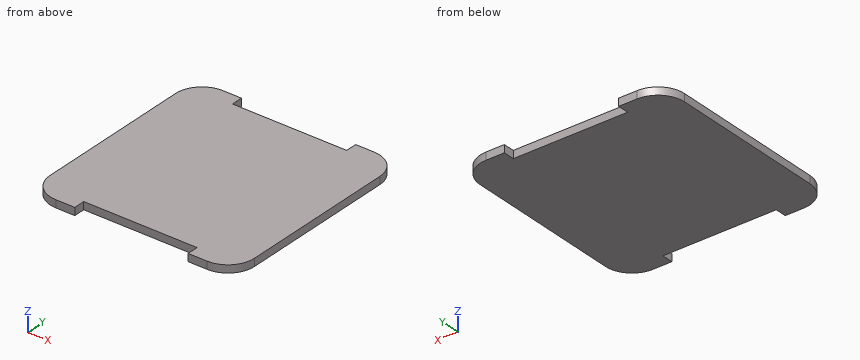
from build123d import *

# Parameters (mm, degrees)
BOSS_EXTRUDE1_DEPTH = 1
CUT_EXTRUDE1_REACH  = 3
SKETCH2_W           = 15.10750805
SKETCH2_H           = 1.5


with BuildPart() as part:
    # Sketch1 → Boss-Extrude1 (new body)
    with BuildSketch(Plane.XY):
        with BuildLine():
            Line((-13.5, 10.5), (-13.5, -10.5))
            ThreePointArc((-13.5, -10.5), (-12.474873734, -12.974873734), (-10, -14))
            Line((-10, -14), (10, -14))
            ThreePointArc((10, -14), (12.474873734, -12.974873734), (13.5, -10.5))
            Line((13.5, -10.5), (13.5, 10.5))
            ThreePointArc((13.5, 10.5), (12.474873734, 12.974873734), (10, 14))
            Line((10, 14), (-10, 14))
            ThreePointArc((-10, 14), (-12.474873734, 12.974873734), (-13.5, 10.5))
        make_face()
    extrude(amount=BOSS_EXTRUDE1_DEPTH)

    # Sketch2 → Cut-Extrude1 (cut, up to next)
    with BuildSketch(Plane.XY.offset(1), mode=Mode.PRIVATE) as cut_extrude1_sk1:
        with Locations((0, 13.25)):
            Rectangle(SKETCH2_W, SKETCH2_H)
    cut_extrude1_tool1 = extrude(cut_extrude1_sk1.sketch, amount=-CUT_EXTRUDE1_REACH, mode=Mode.PRIVATE) & part.part
    add(cut_extrude1_tool1.solids().sort_by_distance((0, 13.25, 1))[0], mode=Mode.SUBTRACT)
    # Sketch2 → Cut-Extrude1 (cut, up to next)
    with BuildSketch(Plane.XY.offset(1), mode=Mode.PRIVATE) as cut_extrude1_sk2:
        Polygon((-7.493203699, -14), (7.493203699, -14), (7.496447466, -12.5), (-7.496447466, -12.5), align=None)
    cut_extrude1_tool2 = extrude(cut_extrude1_sk2.sketch, amount=-CUT_EXTRUDE1_REACH, mode=Mode.PRIVATE) & part.part
    add(cut_extrude1_tool2.solids().sort_by_distance((0, -13.249946, 1))[0], mode=Mode.SUBTRACT)


solid = part.part
The model under review builds one solid part; all positions refer to its coordinate system, in mm. Round coordinates to 2 decimals unless told otherwise and drop trailing zeros. Loops run counter-clockwise (first coordinate to the right, second up) from the corner with the lowest first, then second, coordinate; pieces in that order, holes last. Notation, with made-up numbers: M 70,39 L 93,39 A24 cw 93,51 Z; hole C 50,85.5 d3. An arc over 180 degrees is marked long. Answer as CSV lines item,"result". Start each with the question number.
Item 1: Consider section B-B (x = -1.5). Write out the cut boundary in (y, z).
Item 2: Consider section C-C (y = 12). Write out the cut boundary in (x, z), then the cut area to 3 significant figures.
Item 3: Wall thickness on line 1 (Y direction, x = 0.75, z = 0.3); line 2 (Y direction, x = 10.5, z = 0.4); line 3 (X direction, y = 11.75, z = 0.9): over which ranges is each line inside the solid? List them lowest first. Write a range as [from, to].
Item 4: Consider section A-A (z = 0.65). Write out the cut boundary in (x, y), then the cut area to 3 significant figures.
Answer:
1,outline,"M -12.5,0 L 12.5,0 L 12.5,1 L -12.5,1 Z"
2,outline,"M -13.16,0 L 13.16,0 L 13.16,1 L -13.16,1 Z"
2,area,"26.3 mm^2"
3,line 1,"y = [-12.5, 12.5]"
3,line 2,"y = [-13.96, 13.96]"
3,line 3,"x = [-13.27, 13.27]"
4,outline,"M -13.5,-10.5 A3.5 ccw -10,-14 L -7.49,-14 L -7.5,-12.5 L 7.5,-12.5 L 7.49,-14 L 10,-14 A3.5 ccw 13.5,-10.5 L 13.5,10.5 A3.5 ccw 10,14 L 7.55,14 L 7.55,12.5 L -7.55,12.5 L -7.55,14 L -10,14 A3.5 ccw -13.5,10.5 Z"
4,area,"700 mm^2"
